Source: CAD feature listing. Evaluate the final solid. Frame: model axes, mm. Face numbers are marked on the shaded views. Round coordinates to 2 decimals unless told otherwise and drop trailing zeros. Order: outer loops, then holes, each group sorted by start corner. A loop starts at its lowest first (then second) coordinate and runs counter-clockwise, first axis right, second up. Notation, with made-up numbers: (3.5, 53.25) -> (17.5, 53.25) arc R5 cw to (17.5, 61.25) -> close; hole circle Ø8 at (-25.75, 10). An arc over 180 degrees is marked (long way). Answer as CSV lines item,"result". Start each with the question number.
(1) Section query B-B (y = 8). Count the separate pieces of the cut face and the enclosed holes in it, plus the area to 3 significant figures.
(2) Line query: line 1 along Z through (x, y) = (-7.5, -5); line 2 along Z through (x, y) = (-12, -14); line 3 along X through (y, z) = (12.5, 14). Output: solid intervals per line, ascending. Write a range as from..to.
(3) Section query A-A (y = 30.5). Output: boundary loops of the cut face in (x, z).
(4) Contact query for flat-ended pins moving along their axis: P1, Ø5, axis at y = -47, z = 11, coming from the -X side; P2, Ø5, axis at x = -38.5, z = -15, coming from the -Y side; P3, Ø4, axis at x = -37.5, y = -33, coming from the -Z side. Output: stop coordinate, or through.
(5) Pull-direction query (Y, two-part tool) for the marked faces 1, 2 and 3; classes: +Y half, -Y half, draft (parallel to the pull), parting line (faces both ways), or undercut.
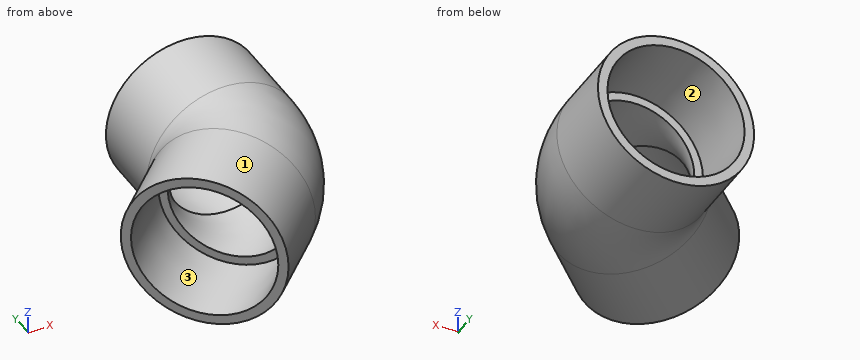
```python
from build123d import *

# Parameters (mm, degrees)
SKETCH3_R   = 34.528125
SKETCH3_R_2 = 26.2509


with BuildPart() as part:
    # Sketch1 → Revolve1 (revolve)
    with BuildSketch(Plane.XY):
        Polygon((-11.505953155, -60.336095813), (13.189751178, -35.64039148), (10.048906599, -32.499546902), (-14.485153123, -57.356895845), align=None)
    revolve(axis=Axis((-35.921024484, -35.921024484, 0), (0.707106781, 0.707106781, 0)))



with BuildPart() as body_2:
    # Sketch2 → Revolve2 (revolve)
    with BuildSketch(Plane.XY):
        Polygon((30.3149, 50.8), (30.0863, 15.875), (34.528125, 15.875), (34.528125, 50.8), align=None)
    revolve(axis=Axis((0, 0, 0), (0, 1, 0)))


with BuildPart() as part_1:
    add(part.part)

    add(body_2.part)  # Sweep1 merges body 2
    # Sweep1: sweep along a path in Sketch4
    with BuildLine(Plane.XY) as sweep1_path:
        ThreePointArc((-11.225320151, -11.225320151), (-2.917365657, 1.208412421), (0, 15.875))
    # Sketch3 → Sweep1 (sweep)
    with BuildSketch(Plane(origin=(-11.225320151, -11.225320151, 0), x_dir=(0, 0, -1), z_dir=(0.707106781, 0.707106781, 0))):
        Circle(SKETCH3_R)
        Circle(SKETCH3_R_2, mode=Mode.SUBTRACT)
    sweep(path=sweep1_path.line)


solid = part_1.part
```
Answer block:
1,separate pieces,"1"
1,enclosed holes,"2"
1,area,"1,670 mm2"
2,line 1,"-34.51..-26.23, 26.23..34.51"
2,line 2,"-34.5..-30.07, 30.07..34.5"
2,line 3,"-32.46..-22.56, 22.11..31.48"
3,outline,"circle Ø69.06 at (0, 0); hole circle Ø60.36 at (0, 0)"
4,P1,"x = -10.04"
4,P2,"y = -4.76"
4,P3,"z = -34.51"
5,face 1,"parting line"
5,face 2,"+Y half"
5,face 3,"undercut"
